Build history of the part. All positions in model axes, mm. A direction names the side the tool comes from. Give positions to 0.01 mm unless a question says otherwise; leave off trailing zeros. Order: outer loops, then holes, each group sorted by start corner. A loop starts at its lowest first (then second) coordinate and runs counter-clockwise, first axis right, second up. Notation, with made-up numbers: (72.5, 84) - (113.5, 84) arc R28 ccw to (113.5, 112) - close; hole circle Ø9 at (0, 58). An arc over 180 degrees is marked (long way). Use a Markdown table: item, result.
from build123d import *

# Parameters (mm, degrees)
F1_DEPTH = 15
F3_DEPTH = 2
F5_DEPTH = 20
F7_DEPTH = 20


with BuildPart() as f1:
    # F0 (on Top) → F1 (new body)
    with BuildSketch(Plane.XY):
        Polygon((-43.4116994914, -2), (-33.3080697806, -2), (-28.2562549252, -10.75), (-33.3080697806, -19.5), (-32.1533692422, -21.5), (-25.9468538484, -10.75), (-27.1015543868, -8.75), (-32.1533692422, 0), (-27.1015543868, 8.75), (-22.0497395314, 8.75), (-16.997924676, 8.75), (-11.9461098206, 0), (-14.4720172483, -4.375), (-16.997924676, -8.75), (-18.1526252144, -10.75), (-15.8432241376, -10.75), (-10.7914092822, -2), (-9.6367087438, 0), (-15.8432241376, 10.75), (-22.0497395314, 10.75), (-28.2562549252, 10.75), (-34.462770319, 0), (-42.2567087438, 0), (-48.4632241376, 10.75), (-54.6697395314, 10.75), (-60.8762549252, 10.75), (-67.082770319, 0), (-74.8767087438, 0), (-81.0832241376, 10.75), (-87.2897395314, 10.75), (-93.4962549252, 10.75), (-99.702770319, 0), (-107.4967087438, 0), (-113.7032241376, 10.75), (-119.9097395314, 10.75), (-126.1162549252, 10.75), (-132.322770319, 0), (-140.1167087438, 0), (-146.3232241376, 10.75), (-152.5297395314, 10.75), (-158.7362549252, 10.75), (-164.942770319, 0), (-175.0464000298, 0), (-181.2529154236, -10.75), (-175.0464000298, -21.5), (-173.8916994914, -19.5), (-178.9435143468, -10.75), (-173.8916994914, -2), (-163.7880697806, -2), (-158.7362549252, -10.75), (-163.7880697806, -19.5), (-162.6333692422, -21.5), (-156.4268538484, -10.75), (-162.6333692422, 0), (-157.5815543868, 8.75), (-152.5297395314, 8.75), (-147.477924676, 8.75), (-142.4261098206, 0), (-148.6329154236, -10.75), (-142.4264000298, -21.5), (-141.2716994914, -19.5), (-146.3235143468, -10.75), (-141.2716994914, -2), (-131.1680697806, -2), (-126.1162549252, -10.75), (-131.1680697806, -19.5), (-130.0133692422, -21.5), (-123.8068538484, -10.75), (-130.0133692422, 0), (-124.9615543868, 8.75), (-119.9097395314, 8.75), (-114.857924676, 8.75), (-109.8061098206, 0), (-116.0129154236, -10.75), (-109.8064000298, -21.5), (-108.6516994914, -19.5), (-113.7035143468, -10.75), (-108.6516994914, -2), (-98.5480697806, -2), (-93.4962549252, -10.75), (-98.5480697806, -19.5), (-97.3933692422, -21.5), (-91.1868538484, -10.75), (-97.3933692422, 0), (-92.3415543868, 8.75), (-87.2897395314, 8.75), (-82.237924676, 8.75), (-77.1861098206, 0), (-83.3929154236, -10.75), (-77.1864000298, -21.5), (-76.0316994914, -19.5), (-81.0835143468, -10.75), (-76.0316994914, -2), (-65.9280697806, -2), (-60.8762549252, -10.75), (-65.9280697806, -19.5), (-64.7733692422, -21.5), (-58.5668538484, -10.75), (-64.7733692422, 0), (-59.7215543868, 8.75), (-54.6697395314, 8.75), (-49.617924676, 8.75), (-44.5661098206, 0), (-50.7729154236, -10.75), (-44.5664000298, -21.5), (-43.4116994914, -19.5), (-48.4635143468, -10.75), align=None)
    extrude(amount=F1_DEPTH)

    # F2 (on face) → F3 (join)
    with BuildSketch(Plane(origin=(0, 0, 0), x_dir=(1, 0, 0), z_dir=(0, 0, -1))):
        Polygon((-32.1533692422, 21.5), (-175.0464000298, 21.5), (-181.2529154236, 10.75), (-175.0464000298, 0), (-158.7362549252, -10.75), (-15.8432241376, -10.75), (-9.6367087438, 0), (-15.8432241376, 10.75), align=None)
    extrude(amount=-F3_DEPTH)

    # F4 (on face) → F5 (join)
    with BuildSketch(Plane.XY.offset(15)):
        Polygon((-11.9461098206, 0), (-18.1526252144, -10.75), (-15.8432241376, -10.75), (-9.6367087438, 0), (-15.8432241376, 10.75), (-28.2562549252, 10.75), (-34.462770319, 0), (-33.3080697806, -2), (-28.2562549252, -10.75), (-25.9468538484, -10.75), (-32.1533692422, 0), (-27.1015543868, 8.75), (-16.997924676, 8.75), align=None)
        Polygon((-43.4116994914, -2), (-42.2567087438, 0), (-48.4632241376, 10.75), (-60.8762549252, 10.75), (-67.082770319, 0), (-65.9280697806, -2), (-60.8762549252, -10.75), (-58.5668538484, -10.75), (-64.7733692422, 0), (-59.7215543868, 8.75), (-49.617924676, 8.75), (-44.5661098206, 0), (-50.7729154236, -10.75), (-48.4635143468, -10.75), align=None)
        Polygon((-76.0316994914, -2), (-74.8767087438, 0), (-81.0832241376, 10.75), (-93.4962549252, 10.75), (-99.702770319, 0), (-98.5480697806, -2), (-93.4962549252, -10.75), (-91.1868538484, -10.75), (-97.3933692422, 0), (-92.3415543868, 8.75), (-82.237924676, 8.75), (-77.1861098206, 0), (-83.3929154236, -10.75), (-81.0835143468, -10.75), align=None)
        Polygon((-108.6516994914, -2), (-107.4967087438, 0), (-113.7032241376, 10.75), (-126.1162549252, 10.75), (-132.322770319, 0), (-131.1680697806, -2), (-126.1162549252, -10.75), (-123.8068538484, -10.75), (-130.0133692422, 0), (-124.9615543868, 8.75), (-114.857924676, 8.75), (-109.8061098206, 0), (-116.0129154236, -10.75), (-113.7035143468, -10.75), align=None)
        Polygon((-141.2716994914, -2), (-140.1167087438, 0), (-146.3232241376, 10.75), (-158.7362549252, 10.75), (-164.942770319, 0), (-158.7362549252, -10.75), (-156.4268538484, -10.75), (-162.6333692422, 0), (-157.5815543868, 8.75), (-147.477924676, 8.75), (-142.4261098206, 0), (-148.6329154236, -10.75), (-146.3235143468, -10.75), align=None)
    extrude(amount=F5_DEPTH)

    # F6 (on face) → F7 (join)
    with BuildSketch(Plane.XY.offset(2)):
        Polygon((-147.477924676, 8.75), (-157.5815543868, 8.75), (-162.6333692422, 0), (-157.5815543868, -8.75), (-147.477924676, -8.75), (-142.4261098206, 0), align=None)
        Polygon((-114.857924676, 8.75), (-124.9615543868, 8.75), (-130.0133692422, 0), (-124.9615543868, -8.75), (-114.857924676, -8.75), (-109.8061098206, 0), align=None)
        Polygon((-82.237924676, 8.75), (-92.3415543868, 8.75), (-97.3933692422, 0), (-92.3415543868, -8.75), (-82.237924676, -8.75), (-77.1861098206, 0), align=None)
        Polygon((-44.6827581202, 0), (-49.7345729756, 8.75), (-59.8382026864, 8.75), (-64.8900175418, 0), (-59.8382026864, -8.75), (-49.7345729756, -8.75), align=None)
        Polygon((-16.8277836429, 8.75), (-26.9314133538, 8.75), (-31.9832282092, 0), (-26.9314133538, -8.75), (-16.8277836429, -8.75), (-11.7759687875, 0), align=None)
    extrude(amount=F7_DEPTH)


solid = f1.part
1) Pin check, flat tips, straight feed: P1, Ø5, axis at x = -21.5, z = 16.5, coming from the -Y side; P2, Ø2.5, axis at x = -72.5, z = 11.5, coming from the +Y side; P3, Ø1.5, axis at y = -17, z = 11, coming from the +X side. Stop position of each tip, or through.
Computed:
| item | result |
|---|---|
| P1 | stops at y = -8.75 |
| P2 | stops at y = 0 |
| P3 | stops at x = -29.12 |
2) Wall check: line 1 (X direction, y = 9.5, z = 27.5); line 2 (Y direction, x = -156, z = 23); line 3 (Z direction, x = -116.5, y = -4). Give the ranges that are in metal, low to high. Write a range as from..to.
Computed:
| item | result |
|---|---|
| line 1 | x = -159.46..-145.6, -126.84..-112.98, -94.22..-80.36, -61.6..-47.74, -28.98..-15.12 |
| line 2 | y = 8.75..10.75 |
| line 3 | z = 0..22 |
3) Tool access for faces 1 (the flat face through (-79, -16, 15)), 2 (the flat face through (-170, 0, 8)), 3 (the flat face through (-71, -2, 8)), 4 (the flat face through (-153, -8.75, 12)): list every direction of +Z, -Z, +X, -X, +Y, -Y with a clear straight run to the whole face (end or side of a thin tool).
Computed:
| item | result |
|---|---|
| face 1 | +Z, +X, -X, -Y |
| face 2 | +Z, -X, +Y |
| face 3 | +Z, -Y |
| face 4 | +Z |
4) Slice it at B-B (z = 19). State how many separate pieces and enclosed holes the cut face has, and give its area (3 significant figures).
Computed:
| item | result |
|---|---|
| separate pieces | 5 |
| enclosed holes | 0 |
| area | 1,910 mm² |
5) Two-plate mould, pull along Y, no slides. Class faces 5 (the flat face through (-47, -16, 15)), 6 (the flat face through (-136, -2, 8)), 7 (the flat face through (-60.94, -6.64, 25.6)): +Y half, -Y half, draft (parallel to the pull), parting line (faces both ways), or undercut.
Computed:
| item | result |
|---|---|
| face 5 | draft |
| face 6 | -Y half |
| face 7 | undercut |
6) Slice it at A-A (x = -137.5). Write the cut outline in (y, z).
Computed:
| item | result |
|---|---|
| outline | (-21.5, 0) - (10.75, 0) - (10.75, 2) - (0, 2) - (0, 15) - (-2, 15) - (-2, 2) - (-21.5, 2) - close |
